```python
from build123d import *

# Parameters (mm, degrees)
F1_DEPTH = 15.875
F2_SIZE  = 1.27
F4_R     = 6.35
F5_DEPTH = 79.375
F6_SIZE  = 5.08


with BuildPart() as f1:
    # F0 (on Front) → F1 (new body)
    with BuildSketch(Plane.XZ):
        Polygon((-1.349322, 10.91544), (-10.127709, 4.289173), (-8.778387, -6.626267), (1.349322, -10.91544), (10.127709, -4.289173), (8.778387, 6.626267), align=None)
    extrude(amount=-F1_DEPTH)

    # F2
    f2_edges = [f1.edges().sort_by_distance(p)[0] for p in [
        (3.714533, 0, 8.770853),
        (-5.738515, 0, 7.602307),
        (-9.453048, 0, -1.168547),
        (-3.714533, 0, -8.770853),
        (5.738515, 0, -7.602307),
        (9.453048, 0, 1.168547),
    ]]
    chamfer(f2_edges, length=F2_SIZE)

    # F4 (on offset) → F5 (join)
    with BuildSketch(Plane(origin=(0, 15.875, 0), x_dir=(1, 0, 0), z_dir=(0, 1, 0))):
        Circle(F4_R)
    extrude(amount=F5_DEPTH)

    # F6
    f6_edges = [f1.edges().sort_by_distance(p)[0] for p in [
        (-6.35, 95.25, 0),
    ]]
    chamfer(f6_edges, length=F6_SIZE)


solid = f1.part
```
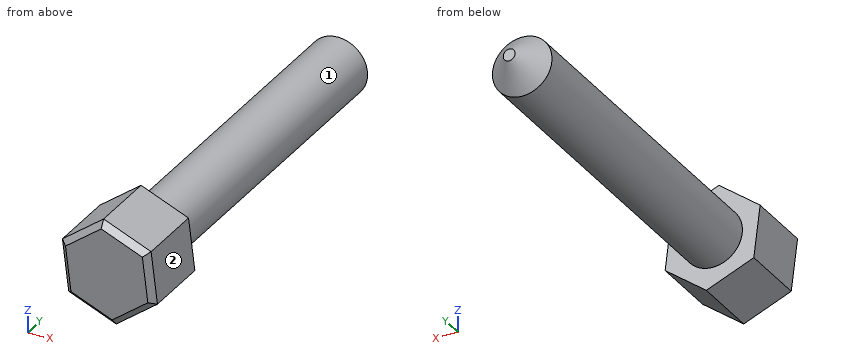
CAD build for the part. Positions are in the model's coordinates, mm. Face numbers are marked on the shaded views. A direction names the side the tool comes from. Round coordinates to 2 decimals unless told otherwise and drop trailing zeros. Order: outer loops, then holes, each group sorted by start corner. A loop starts at its lowest first (then second) coordinate and runs counter-clockwise, first axis right, second up.
Item 1: Saw through at C-C on y = 21. Write the cut outline in (x, z), then the cut area to 3 significant figures.
Item 2: Saw through at B-B on x = 0. Write the cut outline in (y, z) (3 decimals), then the cut area to 3 significant figures.
Item 3: Pin check, flat tips, straight feed: pin 1 (10 mm diameter, centred on y = 71, z = -8.5, fed in from +X); pin 2 (1.5 mm diameter, centred on x = 5, z = -8, fed in from +Y) (3 decimals); pin 3 (3 mm diameter, centred on y = 66.5, z = 6, fed in from +X). Stop position of each tip, or through.
Item 4: Probe line 1 along Z through (x, y) = (0, 63); line 2 along X through (y, z) = (32.5, -0.5); line 3 along Y through (x, z) = (1.25, 0.25). List the from-to ranges inside material, lowest first.
Item 5: Tool access for the marked faces 1 and 2: list every direction of +Z, -Z, +X, -X, +Y, -Y with a clear straight run to the whole face (end or side of a thin tool).
Item 6: Saw through at D-D on z = -7.5. Write the cut outline in (x, y) (3 decimals), then the cut area to 3 significant figures.
Reported:
1. outline: circle Ø12.7 at (0, 0)
1. area: 127 mm2
2. outline: (0, -8.965) - (1.27, -10.344) - (15.875, -10.344) - (15.875, -6.35) - (90.17, -6.35) - (95.25, -1.27) - (95.25, 1.27) - (90.17, 6.35) - (15.875, 6.35) - (15.875, 10.344) - (1.27, 10.344) - (0, 8.965) - close
2. area: 1,310 mm2
3. pin 1: stops at x = 5.3
3. pin 2: stops at y = 15.875
3. pin 3: stops at x = 4.48
4. line 1: z = -6.35 to 6.35
4. line 2: x = -6.33 to 6.33
4. line 3: y = 0 to 95.25
5. face 1: +Y
5. face 2: +Z, +X, +Y, -Y
6. outline: (-6.715, 1.27) - (-3.459, 0) - (3.766, 0) - (5.874, 1.27) - (5.874, 15.875) - (-6.715, 15.875) - close
6. area: 196 mm2
